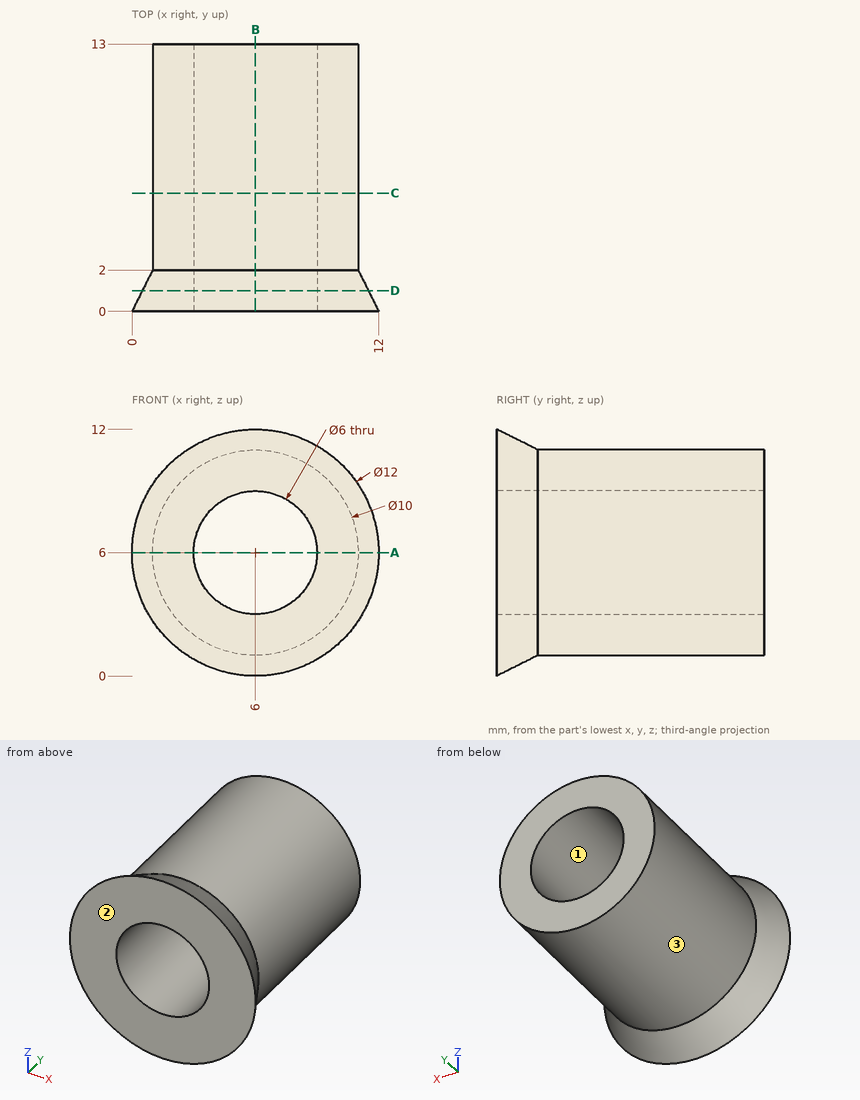
Geometry check sheet. Reference: drawing and pictorial views, mm from the part's lowest x, y, z. Coordinates: 2 decimals unless noted, no trailing zeros. Order: outer loops, then holes, each group sorted by start corner. A loop starts at its lowest first (then second) coordinate and runs counter-clockwise, first axis right, second up. Notation, with made-up numbers: (56, -4) -> (76, -4) arc R18 cw to (76, 0) -> close; hole circle Ø11 at (30, 41). An arc over 180 degrees is marked (long way). Write item = value, one per line. Start each with the question number.
1) Cross-section at C-C (y = 5.75). Enter the section's corners in (x, z).
2) Cross-section at B-B (x = 6). Enter the section's corners in (y, z), then the cut area to 3 significant figures.
3) Material ranges on L1, parallel to X at y = 6.5, z = 6; L2, parallel to X at y = 5, z = 5; L3, parallel to Z at x = 8.5, y = 10.75, recorded low to high.
4) Go/stop test with flat-tipped pins: P1, Ø1, axis at y = 11.5, z = 3.5, coming from the -X side; P2, Ø3, axis at y = 8, z = 8.5, coming from the +X side; P3, Ø4, axis at y = 8.5, z = 7, coming from the +X side; P4, Ø3.5, axis at x = 6, z = 6, coming from the +Y side. Record where each tip stops, or that it passes through.
5) Cross-section at D-D (y = 1). Enter the section's corners in (x, z), then the cut area to 3 significant figures.
6) Mould release check, pull along X, two halves, no side actions. Record for the marked faces 1, 2 and 3: +X half, -X half, draft (parallel to the pull), parting line (faces both ways), or undercut.
7) Cross-section at A-A (z = 6). Enter the section's corners in (x, y), then the cut area to 3 significant figures.
Ans:
q1.outline = circle Ø10 at (6, 6); hole circle Ø6 at (6, 6)
q2.outline = (0, 0) -> (2, 1) -> (13, 1) -> (13, 3) -> (0, 3) -> close; (0, 9) -> (13, 9) -> (13, 11) -> (2, 11) -> (0, 12) -> close
q2.area = 54.0 mm²
q3.L1 = 1 to 3, 9 to 11
q3.L2 = 1.1 to 3.17, 8.83 to 10.9
q3.L3 = 1.67 to 4.34, 7.66 to 10.33
q4.P1 = 1.42
q4.P2 = 10.9
q4.P3 = 11
q4.P4 = through
q5.outline = circle Ø11 at (6, 6); hole circle Ø6 at (6, 6)
q5.area = 66.8 mm²
q6.face_1 = undercut
q6.face_2 = draft
q6.face_3 = parting line
q7.outline = (0, 0) -> (3, 0) -> (3, 13) -> (1, 13) -> (1, 2) -> close; (9, 0) -> (12, 0) -> (11, 2) -> (11, 13) -> (9, 13) -> close
q7.area = 54.0 mm²
